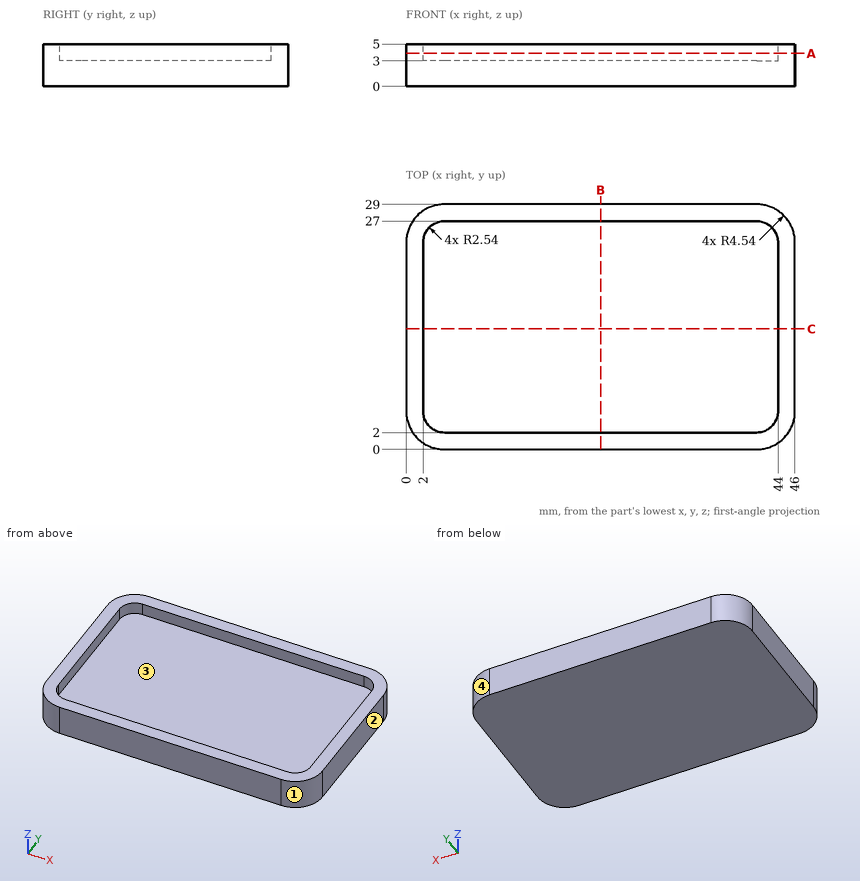
Print and shaded views of the part. All mm, measured from the part's lowest x, y and z. Give positions to 0.01 mm unless a question says otherwise; leave off trailing zeros. Order: outer loops, then holes, each group sorted by start corner. A loop starts at its lowest first (then second) coordinate and runs counter-clockwise, first axis right, second up. Notation, with made-up numbers: (44, 6.5) -> (60, 6.5) arc R23 ccw to (60, 21.5) -> close; hole circle Ø9 at (75.5, 8.25). An arc over 180 degrees is marked (long way). Use CSV: the item, a comma, the result in double quotes.
1. Band-saw the part on B-B, the plane x = 23. Give the cut face in (y, z), then the cut area to 3 significant figures.
Outcome:
outline,"(0, 0) -> (29, 0) -> (29, 5) -> (27, 5) -> (27, 3) -> (2, 3) -> (2, 5) -> (0, 5) -> close"
area,"95.0 mm²"
2. Mould opens along Y. For the marked faces 1, 2, 3 and 4 say: +Y half, -Y half, draft (parallel to the pull), parting line (faces both ways), or undercut.
Outcome:
face 1,"-Y half"
face 2,"draft"
face 3,"undercut"
face 4,"+Y half"
3. Drop a flat-ended pin along its axis: pin 1 (7.5 mm diameter, centred on x = 30, y = 9.5, fed in from +Z). Give the stop position or say it passes through.
Outcome:
pin 1,"z = 3"
4. Band-saw the part on C-C, the plane y = 14.25. Give the cut face in (x, z), then the cut area to 3 significant figures.
Outcome:
outline,"(0, 0) -> (46, 0) -> (46, 5) -> (44, 5) -> (44, 3) -> (2, 3) -> (2, 5) -> (0, 5) -> close"
area,"146 mm²"
5. Drill centre lines: line 1 along X through (y, z) = (12.75, 3.9); line 2 along Y through (x, z) = (6.5, 3.75); line 3 along Z through (x, y) = (42.5, 10.5). Where is each one in solid material? Low to high. Write a range as from..to.
Outcome:
line 1,"0..2, 44..46"
line 2,"0..2, 27..29"
line 3,"0..3"
6. Band-saw the part on A-A, the plane z = 3.9. Give the cut face in (x, y).
Outcome:
outline,"(0, 4.54) arc R4.54 ccw to (4.54, 0) -> (41.46, 0) arc R4.54 ccw to (46, 4.54) -> (46, 24.46) arc R4.54 ccw to (41.46, 29) -> (4.54, 29) arc R4.54 ccw to (0, 24.46) -> close; hole (2, 4.54) arc R2.54 ccw to (4.54, 2) -> (41.46, 2) arc R2.54 ccw to (44, 4.54) -> (44, 24.46) arc R2.54 ccw to (41.46, 27) -> (4.54, 27) arc R2.54 ccw to (2, 24.46) -> close"
